Here's how the part is built. I have some questions about the finished solid (model axes, mm). Face numbers are marked on the shaded views. A direction names the side the tool comes from. Round coordinates to 2 decimals unless told otherwise and drop trailing zeros. Loops run counter-clockwise (first coordinate to the right, second up) from the corner with the lowest first, then second, coordinate; pieces in that order, holes last. Notation, with made-up numbers: M 42,-11 L 88,-11 A21 cw 88,15 Z; hole C 29,74.5 d1. An arc over 180 degrees is marked long. Answer as CSV lines item,"result".
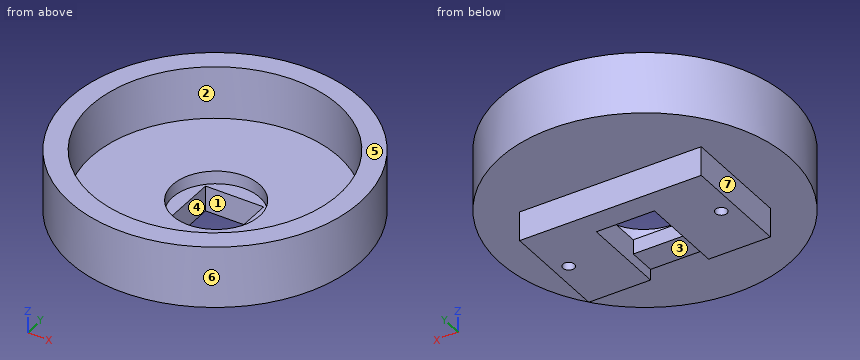
```python
from build123d import *

# Parameters (mm, degrees)
SKETCH1_W                    = 25
SKETCH1_H                    = 15
BOSS_EXTRUDE1_DEPTH          = 4.03
M2_TAPPED_HOLE1_D            = 1.6
M2_TAPPED_HOLE1_DEPTH        = 3
M2_TAPPED_HOLE1_TIP          = 0.480688495
SKETCH5_R                    = 20
BOSS_EXTRUDE2_DEPTH          = 8.5
SKETCH6_R                    = 12.25
CUT_EXTRUDE1_DEPTH           = 5.25
F_1_1_2_6_TAPPED_HOLE1_D     = 34.13252
F_1_1_2_6_TAPPED_HOLE1_DEPTH = 7.25
CUT_EXTRUDE2_DEPTH           = 3.5
SKETCH14_W                   = 8
SKETCH14_H                   = 1.5
CUT_EXTRUDE3_DEPTH           = 13.5
SKETCH15_R                   = 6
CUT_EXTRUDE4_DEPTH           = 13.5


with BuildPart() as part:
    # Sketch1 → Boss-Extrude1 (new body)
    with BuildSketch(Plane.XY):
        with Locations((12.5, 7.5)):
            Rectangle(SKETCH1_W, SKETCH1_H)
    extrude(amount=BOSS_EXTRUDE1_DEPTH)

    # M2 Tapped Hole1
    with Locations(Plane(origin=(0, 0, 0), x_dir=(-1, 0, 0), z_dir=(0, 0, -1))):
        with Locations((-23, 7.5), (-2, 7.5)):
            Hole(M2_TAPPED_HOLE1_D / 2, depth=M2_TAPPED_HOLE1_DEPTH)
            with Locations((0, 0, -(M2_TAPPED_HOLE1_DEPTH + M2_TAPPED_HOLE1_TIP / 2))):  # 118° drill point
                Cone(0, M2_TAPPED_HOLE1_D / 2, M2_TAPPED_HOLE1_TIP, mode=Mode.SUBTRACT)

    # Sketch5 → Boss-Extrude2 (add)
    with BuildSketch(Plane.XY.offset(4.03)):
        with Locations((12.5, 7.5)):
            Circle(SKETCH5_R)
    extrude(amount=BOSS_EXTRUDE2_DEPTH)

    # Sketch6 → Cut-Extrude1 (cut)
    with BuildSketch(Plane.XY.offset(12.53)):
        with Locations((12.5, 7.5)):
            Circle(SKETCH6_R)
    extrude(amount=-CUT_EXTRUDE1_DEPTH, mode=Mode.SUBTRACT)

    # 1-1/2-6 Tapped Hole1
    with Locations(Plane.XY.offset(12.53)):
        with Locations((12.5, 7.5)):
            Hole(F_1_1_2_6_TAPPED_HOLE1_D / 2, depth=F_1_1_2_6_TAPPED_HOLE1_DEPTH)

    # Sketch13 → Cut-Extrude2 (cut)
    with BuildSketch(Plane(origin=(0, 0, 0), x_dir=(-1, 0, 0), z_dir=(0, 0, -1))):
        Polygon((-12.5, 3.75), (-12.5, 7.5), (-12.5, 7.75), (-12.5, 11.75), (-16.5, 11.75), (-16.5, 3.75), align=None)
        Polygon((-12.5, 7.75), (-12.5, 7.5), (-12.5, 3.75), (-8.5, 3.75), (-8.5, 11.75), (-12.5, 11.75), align=None)
    extrude(amount=-CUT_EXTRUDE2_DEPTH, mode=Mode.SUBTRACT)

    # Sketch14 → Cut-Extrude3 (cut)
    with BuildSketch(Plane(origin=(0, 3.75, 0), x_dir=(1, 0, 0), z_dir=(0, 1, 0))):
        with Locations((12.5, -0.75)):
            Rectangle(SKETCH14_W, SKETCH14_H)
    extrude(amount=-CUT_EXTRUDE3_DEPTH, mode=Mode.SUBTRACT)

    # Sketch15 → Cut-Extrude4 (cut)
    with BuildSketch(Plane(origin=(0, 0, 3.5), x_dir=(-1, 0, 0), z_dir=(0, 0, -1))):
        with Locations((-12.5, 7.75)):
            Circle(SKETCH15_R)
    extrude(amount=-CUT_EXTRUDE4_DEPTH, mode=Mode.SUBTRACT)


solid = part.part
```
1. If I drill on line 1 (X direction, y = 7.5, z = 1.15); line 2 (Y direction, x = 12.5, z = 11.25); line 3 (Y direction, x = 12.5, z = 4.65), over which ranges is the centre line in solid material (lowest first)? Write a range as [from, to].
Evaluation:
line 1,"x = [0, 1.2], [2.8, 8.5], [16.5, 22.2], [23.8, 25]"
line 2,"y = [-12.5, -9.57], [24.57, 27.5]"
line 3,"y = [-12.5, 1.75], [13.75, 27.5]"
2. I want a section at A-A, the plane x = 12.5. Please give me the cut outline in (y, z).
Evaluation:
outline,"M -12.5,4.03 L 0,4.03 L 0,1.5 L 3.75,1.5 L 3.75,3.5 L 1.75,3.5 L 1.75,5.28 L -9.57,5.28 L -9.57,12.53 L -12.5,12.53 Z; M 11.75,0 L 15,0 L 15,4.03 L 27.5,4.03 L 27.5,12.53 L 24.57,12.53 L 24.57,5.28 L 13.75,5.28 L 13.75,3.5 L 11.75,3.5 Z"
3. We'd pull the mould along X, two halves only. Please class the marked faces 4, 5, 6 and 7: pulls with the +X half, pulls with the -X half, needs draft (parallel to the pull), parting line crosses it, or undercut.
Evaluation:
face 4,"undercut"
face 5,"needs draft"
face 6,"parting line crosses it"
face 7,"pulls with the -X half"
4. I want a section at D-D, the plane x = 29. Please give me the cut outline in (y, z).
Evaluation:
outline,"M -3.8,4.03 L 18.8,4.03 L 18.8,12.53 L 11.86,12.53 L 11.86,5.28 L 3.14,5.28 L 3.14,12.53 L -3.8,12.53 Z"
5. I want a section at B-B, the plane z = 2. Please give me the cut outline in (x, y).
Evaluation:
outline,"M 0,0 L 25,0 L 25,15 L 0,15 Z; hole C 2,7.5 d1.6; hole M 8.5,3.75 L 16.5,3.75 L 16.5,11.75 L 8.5,11.75 Z; hole C 23,7.5 d1.6"
6. Which directions (+Z, -Z, +X, -X, +Y, -Y) give clear straight access to the entire face, cutting with the end or side of a thin tool? Please do the marked faces 1, 2 and 3.
Evaluation:
face 1,"+Z, -Z"
face 2,"+Z"
face 3,"-Z, -Y"
7. I want a section at C-C, the plane z = 7. Please give me the cut outline in (x, y).
Evaluation:
outline,"C 12.5,7.5 d40; hole C 12.5,7.5 d34.13"
8. For P1, Ø4.5, axis at x = 12, z = 2.5, coming from the -Y side; P2, Ø0.6, axis at x = 11, z = 2.5, coming from the +Y side; P3, Ø2, axis at y = 4.5, z = 1, coming from the +X side, each with a flat end and sliding along its axis, tell me the tip position at first contact or that it passes through.
Evaluation:
P1,"stops at y = -12.5"
P2,"stops at y = 15"
P3,"stops at x = 25"
